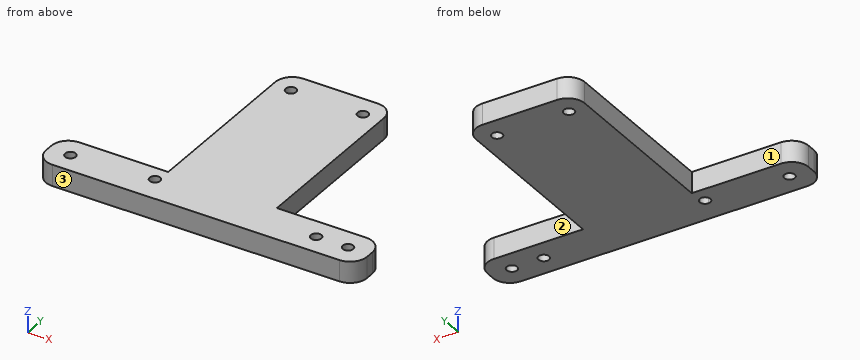
from build123d import *

# Parameters (mm, degrees)
F0_W     = 32.4993
F0_H     = 55.99938
F1_DEPTH = 6.35
F2_R     = 1.5875
F3_DEPTH = 25.4
F4_R     = 5.08
F6_DEPTH = 25.4


with BuildPart() as f1:
    # F0 (on Top) → F1 (new body)
    with BuildSketch(Plane.XY):
        Polygon((-48.424426, 12.7), (-48.424426, 0), (47.574874, 0), (47.574874, 12.7), (15.824874, 12.7), (-16.674426, 12.7), align=None)
        with Locations((-0.424776, 40.69969)):
            Rectangle(F0_W, F0_H)
    extrude(amount=F1_DEPTH)

    # F2 (on face) → F3 (cut)
    with BuildSketch(Plane.XY.offset(6.35)):
        with Locations((41.075014, 6.35)):
            Circle(F2_R)
        with Locations((-41.924566, 6.35)):
            Circle(F2_R)
        with Locations((-11.175326, 62.34938)):
            Circle(F2_R)
        with Locations((10.325774, 62.34938)):
            Circle(F2_R)
    extrude(amount=-F3_DEPTH, mode=Mode.SUBTRACT)

    # F4
    f4_edges = [f1.edges().sort_by_distance(p)[0] for p in [
        (47.574874, 12.7, 3.175),
        (47.574874, 0, 3.175),
        (-48.424426, 0, 3.175),
        (-48.424426, 12.7, 3.175),
        (15.824874, 68.69938, 3.175),
        (-16.674426, 68.69938, 3.175),
    ]]
    fillet(f4_edges, radius=F4_R)

    # F5 (on face) → F6 (cut)
    with BuildSketch(Plane.XY.offset(6.35)):
        with BuildLine():
            ThreePointArc((-16.074986, 7.9375), (-18.785018, 9.060032), (-17.662486, 6.35))
            ThreePointArc((-17.662486, 6.35), (-16.539954, 6.814968), (-16.074986, 7.9375))
        make_face()
        with BuildLine():
            ThreePointArc((29.962514, 6.35), (31.550014, 4.7625), (33.137514, 6.35))
            ThreePointArc((33.137514, 6.35), (31.550014, 7.9375), (29.962514, 6.35))
        make_face()
    extrude(amount=-F6_DEPTH, mode=Mode.SUBTRACT)


solid = f1.part
Work out the finished part from the listing and answer in its coordinate system (mm). Face numbers are marked on the shaded views. A direction names the side the tool comes from. Coordinates: 2 decimals unless noted, no trailing zeros. Write each loop counter-clockwise with the first axis right and the second up, starting at its lowest first coordinate (ties: lowest second). Pieces come first, ordered by that corner, then holes. Notation, with made-up numbers: M 7.5,67.25 L 16.5,67.25 A11 cw 16.5,72.25 Z; hole C 65,72.25 d7. An arc over 180 degrees is marked long. Answer as CSV lines item,"result". Start each with the question number.
Item 1: Section C-C on y = 14.5 is taken. Write down the section's boundary in (x, z), and give its area (3 significant figures).
Item 2: A tool of negligible diameter and unlimited length cuts with its end or side. For the marked faces 1, 2 and 3, from which of +Z, -Z, +X, -X, +Y, -Y can it reach the whole face along a straight path? Write none if from no direction.
Item 3: Consider L1, parallel to Y at x = 41, z = 3; L2, parallel to Y at x = -20, z = 5.5; L3, parallel to X at y = 30, z = 1.75. Determine where each line is inside the solid, lowest interval first.
Item 4: Section A-A on z = 5.25 is taken. Give the number of separate pieces and of enclosed holes in the cut face, and give its area (3 significant figures).
Item 5: Flat-ended cylindrical pins translate along their axes: P1, Ø2, axis at y = 44.5, z = 1, coming from the +X side; P2, Ø4, axis at x = 41.08, y = 6.35, coming from the -Z side; P3, Ø1.9, axis at x = 31.5, z = 4.5, coming from the +Y side; P4, Ø12, axis at x = -23.5, y = 47.5, coming from the +Z side. Find the tip coordinate at first contact, or state that the pin passes through.
Item 6: Section B-B on x = 18.5 is taken. Write down the section's boundary in (y, z), and give its area (3 significant figures).
Checks:
1,outline,"M -16.67,0 L 15.82,0 L 15.82,6.35 L -16.67,6.35 Z"
1,area,"206 mm²"
2,face 1,"+Z, -Z, -X, +Y"
2,face 2,"+Z, -Z, +X, +Y"
2,face 3,"+Z, -Z, +X, -X, -Y"
3,L1,"y = 0 to 4.76, 7.94 to 12.7"
3,L2,"y = 0 to 12.7"
3,L3,"x = -16.67 to 15.82"
4,separate pieces,"1"
4,enclosed holes,"6"
4,area,"2,960 mm²"
5,P1,"stops at x = 15.82"
5,P2,"stops at z = 0"
5,P3,"stops at y = 12.7"
5,P4,"passes through"
6,outline,"M 0,0 L 12.7,0 L 12.7,6.35 L 0,6.35 Z"
6,area,"80.6 mm²"
